Geometry: final body of the model. Coordinates: model frame, mm. Face numbers are marked on the shaded views. Give positions to 0.01 mm unless a question says otherwise; leave off trailing zeros. Write each loop counter-clockwise with the first axis right and the second up, starting at its lowest first coordinate (ties: lowest second). Pieces come first, ordered by that corner, then holes.
Q1. Cut plane C-C on x = 10.5. Return the cut outline in (y, z).
Q2. Cut plane A-A on y = 0. Return the cut outline in (x, z), plus the area to 3 significant figures.
Q3. Line query: L1, parallel to X at y = 0, z = 0.85; L2, parallel to Y at x = 10.5, z = 1.05; L3, parallel to Y at x = 10.5, z = -1.2. Output: solid intervals per line, ascending.
Q4. Cut plane B-B on x = 3.5. Return the cut outline in (y, z).
Q5. Draft query along Y for the marked faces 1, 2 and 3. Return one class per face: pulls with the +Y half, pulls with the -Y half, needs draft (parallel to the pull), parting line crosses it, or undercut.
```python
from build123d import *

# Parameters (mm, degrees)
CUT_EXTRUDE_START   = -3.5
CUT_EXTRUDE_1_DEPTH = 10
SKETCH_3_W          = 4
SKETCH_3_H          = 19.670556204
CUT_EXTRUDE_2_DEPTH = 10
CUT_EXTRUDE_START_2 = -29
SKETCH_4_R          = 4
SKETCH_4_R_2        = 2
CUT_EXTRUDE_3_DEPTH = 29
SKETCH_5_R          = 1
CUT_EXTRUDE_4_DEPTH = 5
CHAMFER_1_SIZE      = 0.25


with BuildPart() as part:
    # 草图1 → 旋转2 (revolve)
    with BuildSketch(Plane.XY, mode=Mode.PRIVATE) as revolve_2_sk:
        Polygon((0, 2), (0, 0), (17, 0), (21, 0), (21, 2), (17, 2), (17, 4), (4, 4), (4, 2), align=None)
    revolve(revolve_2_sk.sketch.rotate(Axis((-16.701754386, 0, 0), (1, 0, 0)), 180), axis=Axis((-16.701754386, 0, 0), (1, 0, 0)))

    # 草图2 → 切除-拉伸1 (cut)
    with BuildSketch(Plane.XY.offset(CUT_EXTRUDE_START)):
        Polygon((12.5, -5.827233832), (12.5, 4), (10.5, 4), (8.5, 4), (8.5, -5.827233832), align=None)
    extrude(amount=-CUT_EXTRUDE_1_DEPTH, mode=Mode.SUBTRACT)

    # 草图3 → 切除-拉伸2 (cut)
    with BuildSketch(Plane(origin=(0, 0, 0), x_dir=(1, 0, 0), z_dir=(0, 1, 0)).offset(CUT_EXTRUDE_START)):
        with Locations((10.5, 3.5)):
            Rectangle(SKETCH_3_W, SKETCH_3_H)
    extrude(amount=-CUT_EXTRUDE_2_DEPTH, mode=Mode.SUBTRACT)

    # 草图4 → 切除-拉伸3 (cut)
    with BuildSketch(Plane(origin=(21, 0, 0), x_dir=(0, 0, -1), z_dir=(1, 0, 0)).offset(CUT_EXTRUDE_START_2)):
        Circle(SKETCH_4_R)
        with Locations(Location((0, 0, 0), (0, 0, 270))):
            Circle(SKETCH_4_R_2, mode=Mode.SUBTRACT)
    extrude(amount=CUT_EXTRUDE_3_DEPTH, mode=Mode.SUBTRACT)

    # 草图5 → 切除-拉伸4 (cut, symmetric)
    with BuildSketch(Plane.XY):
        with Locations((10.5, 0)):
            Circle(SKETCH_5_R)
    extrude(amount=CUT_EXTRUDE_4_DEPTH, both=True, mode=Mode.SUBTRACT)

    # 倒角1
    chamfer_1_edges = [part.edges().sort_by_distance(p)[0] for p in [
        (0, 2, 0),
        (21, 2, 0),
    ]]
    chamfer(chamfer_1_edges, length=CHAMFER_1_SIZE)


solid = part.part
```
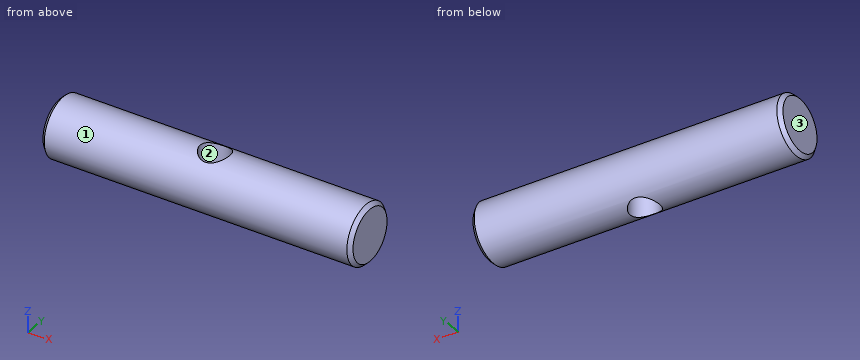
Data:
1. outline: (-1, -1.73) - (-1, 1.73) arc R2 ccw to start; (1, -1.73) arc R2 ccw to (1, 1.73) - close
2. outline: (0, -1.75) - (0.25, -2) - (9.5, -2) - (9.5, 2) - (0.25, 2) - (0, 1.75) - close; (11.5, -2) - (20.75, -2) - (21, -1.75) - (21, 1.75) - (20.75, 2) - (11.5, 2) - close
2. area: 75.9 mm2
3. L1: x = 0 to 9.5, 11.5 to 21
3. L2: y = -1.7 to -1, 1 to 1.7
3. L3: y = -1.6 to -1, 1 to 1.6
4. outline: circle Ø4 at (0, 0)
5. face 1: parting line crosses it
5. face 2: undercut
5. face 3: needs draft
